Could you check a few things on this drawing? It's one solid part, dimensions in mm from its lowest x, y, z. Coordinates: 2 decimals unless noted, no trailing zeros. Order: outer loops, then holes, each group sorted by start corner. A loop starts at its lowest first (then second) coordinate and runs counter-clockwise, first axis right, second up. Notation, with made-up numbers: (58.5, 11) -> (75.5, 11) arc R9 ccw to (75.5, 21) -> close; hole circle Ø6 at (61, 24.25). An arc over 180 degrees is marked (long way). Answer as CSV lines item,"result".
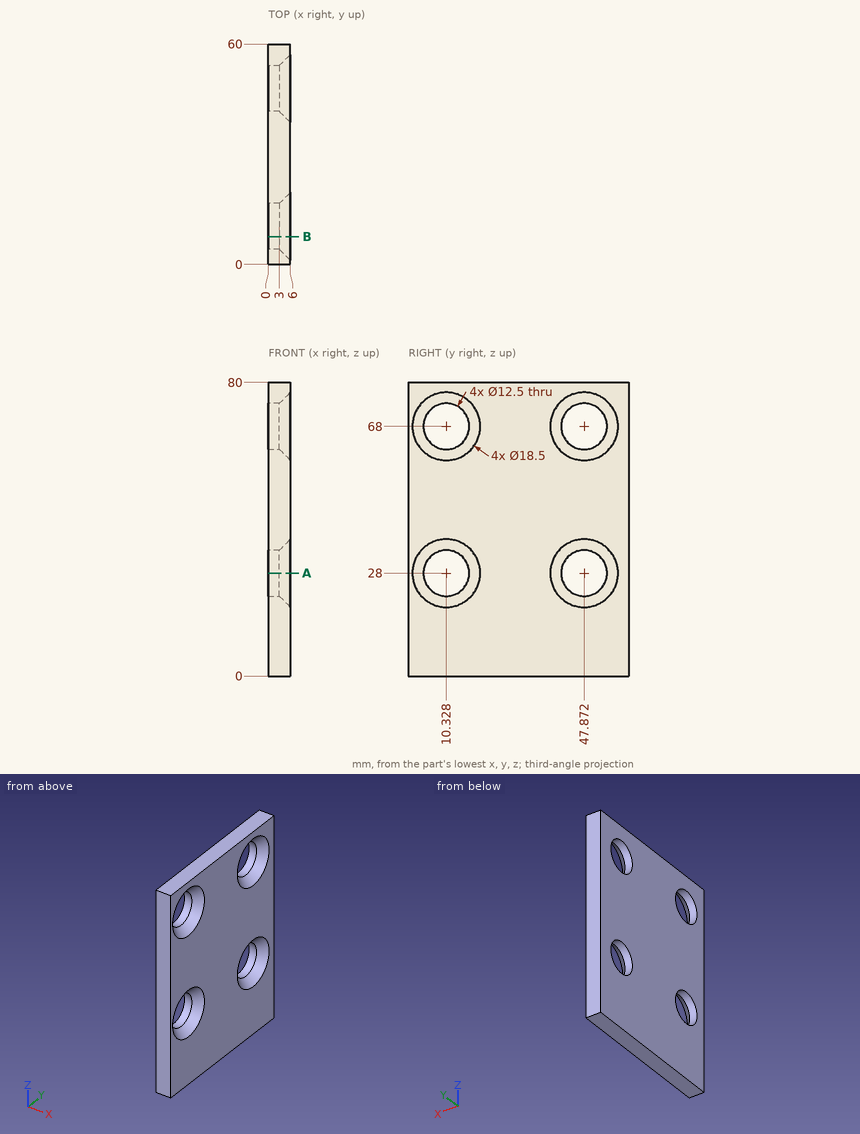
Q1. Imagine slicing it at B-B (y = 7.5). Give the number of separate pieces and of enclosed holes in the cut face, and give its area (3 significant figures).
Solution:
separate pieces,"3"
enclosed holes,"0"
area,"327 mm2"
Q2. If I drill on line 1 (Y direction, x = 0.9, z = 28); line 2 (Z direction, x = 2.9, y = 15); line 3 (Z direction, x = 5.45, y = 5), over which ranges is the centre line in solid material (lowest first)?
Solution:
line 1,"0 to 4.08, 16.58 to 41.62, 54.12 to 60"
line 2,"0 to 23.85, 32.15 to 63.85, 72.15 to 80"
line 3,"0 to 21.12, 34.88 to 61.12, 74.88 to 80"
Q3. For P1, Ø10, axis at y = 33, z = 15.5, coming from the -X side, with a flat end and sliding along its axis, tell me the tip position at first contact or that it passes through.
Solution:
P1,"x = 0"
Q4. Imagine slicing it at A-A (z = 28). List the corners of the cut face in (x, y) for me.
Solution:
outline,"(0, 0) -> (6, 0) -> (6, 1.08) -> (3, 4.08) -> (0, 4.08) -> close; (0, 16.58) -> (3, 16.58) -> (6, 19.58) -> (6, 38.62) -> (3, 41.62) -> (0, 41.62) -> close; (0, 54.12) -> (3, 54.12) -> (6, 57.12) -> (6, 60) -> (0, 60) -> close"
